Source: CAD feature listing. Evaluate the final solid. Frame: model axes, mm. A direction names the side the tool comes from. Round coordinates to 2 decimals unless told otherwise and drop trailing zeros. Loops run counter-clockwise (first coordinate to the right, second up) from the corner with the lowest first, then second, coordinate; pieces in that order, holes last. Notation, with made-up numbers: (37, 75) - (59, 75) arc R19 cw to (59, 95) - close; hole circle Ø4 at (44, -29.5). An arc over 180 degrees is marked (long way). One line per question, with ' | ' between items. Start each with the question number.
1. Ray query, line 1 (X direction, y = 2.25, z = 2.25); line 2 (X direction, y = 2, z = -3.25); line 3 (Z direction, x = 62.5, y = 3.75). Return the intervals inside material, ascending.
2. Mould query, pull axis X, two halves, no side actions, for faces 1 (the flat face through (56, 8.35, 3)), 2 (the flat face through (22, 3, -20.4)), 3 (the flat face through (-31.086, 0, 3)). Classes: pulls with the +X half, pulls with the -X half, needs draft (parallel to the pull), parting line crosses it, or undercut.
3. Pin query (flat end, axial travel): pin 1 (6 mm diameter, centred on y = 6, z = -16, fed in from -X); pin 2 (13.5 mm diameter, centred on y = 1, z = -9, fed in from +X); pin 3 (7 mm diameter, centred on x = 64, y = -6, fed in from -Z). Return the tip coordinate at first contact, or that it passes through.
4. Access query for faces 4 (the flat face through (-8.086, 3, -7)), 5 (the flat face through (-17, 8.35, 3)), 6 (the flat face through (-22, 9, 0)), 7 (the flat face through (67, 0, 0)), 8 (the flat face through (-29, -8.32, 3)). Directions: +Z, -Z, +X, -X, +Y, -Y. A direction counts if a zero-diameter tool reaches every point of the face in a straight line with its end or side. Return the directions, or none.
5. Cut plane A-A (y = -6.25). Return loops of the section in (x, z), then the cut area to 3 significant figures.
6. Cut plane D-D (z = -8). Return loops of the section in (x, y), then the cut area to 3 significant figures.
7. Cut plane B-B (y = 2.75). Return loops of the section in (x, z), then the cut area to 3 significant figures.
8. Cut plane C-C (x = 70). Return loops of the section in (y, z).
```python
from build123d import *

# Parameters (mm, degrees)
F0_W     = 60.5
F0_H     = 6.85
F1_DEPTH = 5.25
F2_DEPTH = 20.4
F3_W     = 60.5
F3_H     = 20.4
F4_DEPTH = 3
F5_DEPTH = 7
F6_DEPTH = 14
F7_DEPTH = 7.1
F8_DEPTH = 5.25
F9_DEPTH = 0.25


with BuildPart() as f1:
    # F0 (on Top) → F1 (new body)
    with BuildSketch(Plane.XY):
        with BuildLine():
            Line((71.054384552, 12), (70.0535051376, 12))
            Line((70.0535051376, 12), (60.4137502015, 12))
            Line((60.4137502015, 12), (60.4137502015, 8.35))
            Line((60.4137502015, 8.35), (60.4137502015, -12))
            Line((60.4137502015, -12), (76.9137502015, -12))
            Line((76.9137502015, -12), (76.9137502015, 5.3627402522))
            Line((76.9137502015, 5.3627402522), (76.9137502015, 5.9437831573))
            ThreePointArc((76.9137502015, 5.9437831573), (75.1294427626, 10.0800376979), (71.054384552, 12))
        make_face()
        with BuildLine():
            Line((-26.0862497985, -8.32), (-26.0862497985, 8.35))
            Line((-26.0862497985, 8.35), (-26.0862497985, 12))
            ThreePointArc((-26.0862497985, 12), (-29.3762488381, 10.7847383112), (-31.0862497985, 7.7225738205))
            Line((-31.0862497985, 7.7225738205), (-31.0862497985, -8.32))
            Line((-31.0862497985, -8.32), (-26.0862497985, -8.32))
        make_face()
        Polygon((60.4137502015, 8.35), (60.4137502015, 12), (52.4137502015, 12), (-8.0862497985, 12), (-26.0862497985, 12), (-26.0862497985, 8.35), align=None)
        with Locations((22.1637502015, 15.425)):
            Rectangle(F0_W, F0_H)
    extrude(amount=F1_DEPTH)

    # F0 (on Top) → F2 (join)
    with BuildSketch(Plane.XY):
        with Locations((22.1637502015, 15.425)):
            Rectangle(F0_W, F0_H)
    extrude(amount=-F2_DEPTH)

    # F3 (on face) → F4 (join)
    with BuildSketch(Plane.XZ.offset(-12)):
        with Locations((22.1637502015, -10.2)):
            Rectangle(F3_W, F3_H)
    extrude(amount=F4_DEPTH)

    # F5 (add): a face of the model
    f5_faces = [f1.faces().sort_by_distance(p)[0] for p in [
        (22.1637502015, 18.85, -7.575),
    ]]
    extrude(f5_faces, amount=-F5_DEPTH)

    # F6 (add): a face of the model
    f6_faces = [f1.faces().sort_by_distance(p)[0] for p in [
        (22.1637502015, 9, -10.2),
    ]]
    extrude(f6_faces, amount=F6_DEPTH)

    # F7 (cut): a face of the model
    f7_faces = [f1.faces().sort_by_distance(p)[0] for p in [
        (22.1637502015, 18.85, -7.575),
    ]]
    extrude(f7_faces, amount=-F7_DEPTH, mode=Mode.SUBTRACT)

    # F8 (add): a face of the model
    f8_faces = [f1.faces().sort_by_distance(p)[0] for p in [
        (22.1637502015, 1.675, 0),
    ]]
    extrude(f8_faces, amount=F8_DEPTH)

    # F9 (add): a face of the model
    f9_faces = [f1.faces().sort_by_distance(p)[0] for p in [
        (22.1637502015, 11.75, -7.575),
    ]]
    extrude(f9_faces, amount=F9_DEPTH)


solid = f1.part
```
Answers follow:
1) line 1: x = -31.09 to -26.09, -8.09 to 52.41, 60.41 to 76.91 | line 2: x = -8.09 to 52.41 | line 3: z = 0 to 5.25
2) face 1: undercut | face 2: needs draft | face 3: pulls with the -X half
3) pin 1: stops at x = -8.09 | pin 2: stops at x = 52.41 | pin 3: stops at z = 0
4) face 4: -Z, -Y | face 5: +Z, -Z, -Y | face 6: -Z, -X, +Y, -Y | face 7: -Z, +X, +Y, -Y | face 8: +Z, -Z, -X, -Y
5) outline: (-31.09, 0) - (-26.09, 0) - (-26.09, 5.25) - (-31.09, 5.25) - close; (60.41, 0) - (76.91, 0) - (76.91, 5.25) - (60.41, 5.25) - close | area: 113 mm2
6) outline: (-8.09, -5) - (52.41, -5) - (52.41, 12) - (-8.09, 12) - close | area: 1,030 mm2
7) outline: (-31.09, 0) - (-26.09, 0) - (-26.09, 5.25) - (-31.09, 5.25) - close; (-8.09, -20.4) - (52.41, -20.4) - (52.41, 5.25) - (-8.09, 5.25) - close; (60.41, 0) - (76.91, 0) - (76.91, 5.25) - (60.41, 5.25) - close | area: 1,660 mm2
8) outline: (-12, 0) - (12, 0) - (12, 5.25) - (-12, 5.25) - close
